from build123d import *

# Parameters (mm, degrees)
BOSS_EXTRUDE1_DEPTH                                 = 6
BOSS_EXTRUDE2_START                                 = -6
BOSS_EXTRUDE2_DEPTH                                 = 6
CBORE_FOR_M3_HEX_SOCKET_HEAD_CAP_SCREW1_D           = 3.4
CBORE_FOR_M3_HEX_SOCKET_HEAD_CAP_SCREW1_CBORE_D     = 6.5
CBORE_FOR_M3_HEX_SOCKET_HEAD_CAP_SCREW1_CBORE_DEPTH = 3.4
CBORE_FOR_M3_HEX_SOCKET_HEAD_CAP_SCREW2_D           = 3.4
CBORE_FOR_M3_HEX_SOCKET_HEAD_CAP_SCREW2_DEPTH       = 10
CBORE_FOR_M3_HEX_SOCKET_HEAD_CAP_SCREW2_CBORE_D     = 6.5
CBORE_FOR_M3_HEX_SOCKET_HEAD_CAP_SCREW2_CBORE_DEPTH = 3.4
CBORE_FOR_M3_HEX_SOCKET_HEAD_CAP_SCREW2_TIP         = 1.021463052
CUT_EXTRUDE1_REACH                                  = 162.125
SKETCH8_W                                           = 76
SKETCH8_H                                           = 78
CUT_EXTRUDE1_DIRECTION_2_DEPTH                      = 161.12495121
FILLET2_R                                           = 5


with BuildPart() as part:
    # Sketch1 → Boss-Extrude1 (new body)
    with BuildSketch(Plane.XY):
        with BuildLine():
            Line((-30, 0), (-30, 152))
            Line((-30, 152), (30, 152))
            Line((30, 152), (30, 0))
            ThreePointArc((30, 0), (0, -30), (-30, 0))
        make_face()
    extrude(amount=BOSS_EXTRUDE1_DEPTH)

    # Sketch7 → Boss-Extrude2 (add)
    with BuildSketch(Plane.XY.offset(6).offset(BOSS_EXTRUDE2_START)):
        with BuildLine():
            Line((-50, 152), (-50, 32))
            Line((-50, 32), (-26.72417541, -13.631524078))
            ThreePointArc((-26.72417541, -13.631524078), (-29.169549725, -7.009805194), (-30, 0))
            Line((-30, 0), (-30, 32))
            Line((-30, 32), (-30, 152))
            Line((-30, 152), (-50, 152))
        make_face()
        with BuildLine():
            ThreePointArc((30, 0), (29.169549725, -7.009805194), (26.72417541, -13.631524078))
            Line((26.72417541, -13.631524078), (50, 32))
            Line((50, 32), (50, 152))
            Line((50, 152), (30, 152))
            Line((30, 152), (30, 32))
            Line((30, 32), (30, 0))
        make_face()
    extrude(amount=BOSS_EXTRUDE2_DEPTH)

    # CBORE for M3 Hex Socket Head Cap Screw1 (through all)
    with Locations(Plane.XY.offset(6)):
        with Locations((-17.67766953, 17.67766953), (0, 25), (17.67766953, 17.67766953), (25, 0), (17.67766953, -17.67766953), (0, -25), (-17.67766953, -17.67766953), (-25, 0)):
            CounterBoreHole(CBORE_FOR_M3_HEX_SOCKET_HEAD_CAP_SCREW1_D / 2, CBORE_FOR_M3_HEX_SOCKET_HEAD_CAP_SCREW1_CBORE_D / 2, CBORE_FOR_M3_HEX_SOCKET_HEAD_CAP_SCREW1_CBORE_DEPTH)

    # CBORE for M3 Hex Socket Head Cap Screw2
    with Locations(Plane(origin=(0, 0, 0), x_dir=(-1, 0, 0), z_dir=(0, 0, -1))):
        with Locations((-40, 149), (0, 35), (20, 35), (40, 35), (-20, 35), (-40, 35), (0, 149), (20, 149), (40, 149), (-20, 149)):
            CounterBoreHole(CBORE_FOR_M3_HEX_SOCKET_HEAD_CAP_SCREW2_D / 2, CBORE_FOR_M3_HEX_SOCKET_HEAD_CAP_SCREW2_CBORE_D / 2, CBORE_FOR_M3_HEX_SOCKET_HEAD_CAP_SCREW2_CBORE_DEPTH, depth=CBORE_FOR_M3_HEX_SOCKET_HEAD_CAP_SCREW2_DEPTH)
            with Locations((0, 0, -(CBORE_FOR_M3_HEX_SOCKET_HEAD_CAP_SCREW2_DEPTH + CBORE_FOR_M3_HEX_SOCKET_HEAD_CAP_SCREW2_TIP / 2))):  # 118° drill point
                Cone(0, CBORE_FOR_M3_HEX_SOCKET_HEAD_CAP_SCREW2_D / 2, CBORE_FOR_M3_HEX_SOCKET_HEAD_CAP_SCREW2_TIP, mode=Mode.SUBTRACT)

    # Sketch8 → Cut-Extrude1 (cut, up to next)
    with BuildSketch(Plane(origin=(0, 0, 0), x_dir=(-1, 0, 0), z_dir=(0, 0, -1)), mode=Mode.PRIVATE) as cut_extrude1_sk1:
        with Locations((0, 93)):
            Rectangle(SKETCH8_W, SKETCH8_H)
    cut_extrude1_tool1 = extrude(cut_extrude1_sk1.sketch, amount=-CUT_EXTRUDE1_REACH, mode=Mode.PRIVATE) & part.part
    add(cut_extrude1_tool1.solids().sort_by_distance((0, 93, 0))[0], mode=Mode.SUBTRACT)

    # Sketch8 → Cut-Extrude1 direction 2 (cut)
    with BuildSketch(Plane(origin=(0, 0, 0), x_dir=(-1, 0, 0), z_dir=(0, 0, -1))):
        with Locations((0, 93)):
            Rectangle(SKETCH8_W, SKETCH8_H)
    extrude(amount=CUT_EXTRUDE1_DIRECTION_2_DEPTH, mode=Mode.SUBTRACT)

    # Fillet2
    fillet2_edges = [part.edges().sort_by_distance(p)[0] for p in [
        (38, 132, 3),
        (38, 54, 3),
        (-38, 54, 3),
        (-38, 132, 3),
    ]]
    fillet(fillet2_edges, radius=FILLET2_R)


solid = part.part
Read the model definition and answer for the solid it produces. Units are mm, in the model's axes. A direction names the side the tool comes from. Round coordinates to 2 decimals unless told otherwise and drop trailing zeros. Write each loop counter-clockwise with the first axis right and the second up, starting at its lowest first coordinate (ties: lowest second). Pieces come first, ordered by that corner, then holes. Notation, with made-up numbers: M 18,-29 L 60,-29 A14 ccw 60,-22 Z; hole C -21.5,63.25 d8. An arc over 180 degrees is marked long. Use a Markdown table: item, result.
1) The part is cut by section B-B (y = 25). Write down the section's boundary in (x, z), plus the area to 3 significant figures.
Answers follow:
| item | result |
|---|---|
| outline | M -46.43,0 L -1.7,0 L -1.7,2.6 L -3.25,2.6 L -3.25,6 L -46.43,6 Z; M 1.7,0 L 46.43,0 L 46.43,6 L 3.25,6 L 3.25,2.6 L 1.7,2.6 Z |
| area | 526 mm2 |
2) For a pull along X with two mould halves and no side action, classify faces 4 (the flat face through (1, 152, 4)), 5 (the cylindrical face through (-0.37, 33.34, 4.72)), 6 (the flat face through (38.199, 8.865, 2.958)) as pulls with the +X half, pulls with the -X half, needs draft (parallel to the pull), parting line crosses it, or undercut.
Answers follow:
| item | result |
|---|---|
| face 4 | needs draft |
| face 5 | undercut |
| face 6 | pulls with the +X half |
3) Straight lines are drawn through the part: line 1 along X through (y, z) = (149, 4.1); line 2 along X through (y, z) = (97, 5.1); line 3 along Y through (x, z) = (-26.5, 2.4). For each, find the intervals that lie inside material, in ascending order. Write a range as [from, to].
Answers follow:
| item | result |
|---|---|
| line 1 | x = [-50, -41.7], [-38.3, -21.7], [-18.3, -1.7], [1.7, 18.3], [21.7, 38.3], [41.7, 50] |
| line 2 | x = [-50, -38], [38, 50] |
| line 3 | y = [-14.06, -0.8], [0.8, 54], [132, 152] |
4) The part is cut by section C-C (z = 4.35). Give the number of separate pieces and of enclosed holes in the cut face, plus the area to 3 significant figures.
Answers follow:
| item | result |
|---|---|
| separate pieces | 1 |
| enclosed holes | 19 |
| area | 9,860 mm2 |
5) Flat-ended cylindrical pins translate along their axes: pin 1 (3 mm diameter, centred on x = -20, y = 149, fed in from -Z); pin 2 (2 mm diameter, centred on x = 0.5, y = 26.5, fed in from +Z); pin 3 (3 mm diameter, centred on x = -9, z = 1, fed in from -Y); pin 4 (4 mm diameter, centred on x = 20, y = 149, fed in from -Z). Find the tip coordinate at first contact, or state that the pin passes through.
Answers follow:
| item | result |
|---|---|
| pin 1 | passes through |
| pin 2 | stops at z = 2.6 |
| pin 3 | stops at y = -29.05 |
| pin 4 | stops at z = 3.4 |
6) The part is cut by section D-D (x = -30.5). Write down the section's boundary in (y, z).
Answers follow:
| item | result |
|---|---|
| outline | M -6.23,0 L 54,0 L 54,6 L -6.23,6 Z; M 132,0 L 152,0 L 152,6 L 132,6 Z |
7) A tool of negligible diameter and unlimited length cuts with its end or side. For faces 1 (the flat face through (-38, 93, 3)), 2 (the cylindrical face through (21.753, 0.143, 4.324)), 3 (the flat face through (-21.4, 33.6, 3.4)), from which of +Z, -Z, +X, -X, +Y, -Y can it reach the whole face along a straight path? Write none if from no direction.
Answers follow:
| item | result |
|---|---|
| face 1 | +Z, -Z |
| face 2 | +Z |
| face 3 | -Z |
8) The part is cut by section A-A (x = 5). Write down the section's boundary in (y, z), plus the area to 3 significant figures.
Answers follow:
| item | result |
|---|---|
| outline | M -29.58,0 L 54,0 L 54,6 L -29.58,6 Z; M 132,0 L 152,0 L 152,6 L 132,6 Z |
| area | 621 mm2 |
